from build123d import *

# Parameters (mm, degrees)
SKETCH_1_W          = 110
SKETCH_1_H          = 85.2
EXTRUDE_1_DEPTH     = 4
SKETCH_2_W          = 83
SKETCH_2_H          = 11
CUT_EXTRUDE_1_DEPTH = 4
SKETCH_3_R          = 1.6
CUT_EXTRUDE_2_DEPTH = 4
FILLET_1_R          = 2


with BuildPart() as part:
    # 草图1 → 凸台-拉伸1 (new body)
    with BuildSketch(Plane(origin=(0, 0, 0), x_dir=(1, 0, 0), z_dir=(0, 1, 0))):
        Rectangle(SKETCH_1_W, SKETCH_1_H)
    extrude(amount=EXTRUDE_1_DEPTH)

    # 草图2 → 切除-拉伸1 (cut)
    with BuildSketch(Plane(origin=(0, 4, 0), x_dir=(1, 0, 0), z_dir=(0, 1, 0))):
        with Locations((-55, -42.6)):
            Rectangle(SKETCH_2_W, SKETCH_2_H)
        with Locations((55, -42.6)):
            Rectangle(SKETCH_2_W, SKETCH_2_H)
        with Locations((55, 42.6)):
            Rectangle(SKETCH_2_W, SKETCH_2_H)
        with Locations((-55, 42.6)):
            Rectangle(SKETCH_2_W, SKETCH_2_H)
    extrude(amount=-CUT_EXTRUDE_1_DEPTH, mode=Mode.SUBTRACT)

    # 草图3 → 切除-拉伸2 (cut)
    with BuildSketch(Plane(origin=(0, 4, 0), x_dir=(1, 0, 0), z_dir=(0, 1, 0))):
        with Locations(Location((-8, -39.85, 0), (0, 0, 270))):
            Circle(SKETCH_3_R)
        with Locations(Location((8, -39.85, 0), (0, 0, 90))):
            Circle(SKETCH_3_R)
        with Locations(Location((8, 39.85, 0), (0, 0, 270))):
            Circle(SKETCH_3_R)
        with Locations(Location((-8, 39.85, 0), (0, 0, 90))):
            Circle(SKETCH_3_R)
    extrude(amount=-CUT_EXTRUDE_2_DEPTH, mode=Mode.SUBTRACT)

    # 圆角1
    fillet_1_edges = [part.edges().sort_by_distance(p)[0] for p in [
        (-13.5, 2, 42.6),
        (-13.5, 2, 37.1),
        (-55, 2, 37.1),
        (13.5, 2, 42.6),
        (55, 2, 37.1),
        (13.5, 2, 37.1),
        (55, 2, -37.1),
        (13.5, 2, -42.6),
        (13.5, 2, -37.1),
        (-13.5, 2, -42.6),
        (-55, 2, -37.1),
        (-13.5, 2, -37.1),
    ]]
    fillet(fillet_1_edges, radius=FILLET_1_R)


solid = part.part
The model under review builds one solid part; all positions refer to its coordinate system, in mm. A direction names the side the tool comes from. Coordinates: 2 decimals unless noted, no trailing zeros. Loops run counter-clockwise (first coordinate to the right, second up) from the corner with the lowest first, then second, coordinate; pieces in that order, holes last.
(1) Draft analysis for pull direction Z (two halves, no side actions). For faces 5 (the cylindrical face through (-9.56, 2.03, 39.5)), 6 (the flat face through (0, 2, -42.6)), 7 (the flat face through (0, 2, 42.6)), 8 (the flat face through (-1, 4, -1)), state which applies: +Z half, -Z half, draft (parallel to the pull), parting line (faces both ways), or undercut.
Determined:
face 5: undercut
face 6: -Z half
face 7: +Z half
face 8: draft
(2) Tool access review of faces 1 (the flat face through (-35, 2, 37.1)), 2 (the flat face through (-35, 2, -37.1)), 3 (the flat face through (34, 2, 37.1)), 4 (the flat face through (34, 2, -37.1)): name each direction out of +Z, -Z, +X, -X, +Y, -Y from which nothing blocks a thin tool from reaching the whole face with its end or side.
Determined:
face 1: +Z, -X, +Y, -Y
face 2: -Z, -X, +Y, -Y
face 3: +Z, +X, +Y, -Y
face 4: -Z, +X, +Y, -Y
(3) Consider section A-A, the plane x = 8. Give the boundary of the cut face in (y, z), plus the area to 3 significant figures.
Determined:
outline: (0, -42.6) - (4, -42.6) - (4, -41.45) - (0, -41.45) - close; (0, -38.25) - (4, -38.25) - (4, 38.25) - (0, 38.25) - close; (0, 41.45) - (4, 41.45) - (4, 42.6) - (0, 42.6) - close
area: 315 mm2
(4) Consider section C-C, the plane x = -28. Give the boundary of the cut face in (y, z), plus the area to 3 significant figures.
Determined:
outline: (0, -37.1) - (4, -37.1) - (4, 37.1) - (0, 37.1) - close
area: 297 mm2
(5) Consider section B-B, the plane y = 1.45. Give the boundary of the cut face in (x, z), plus the area to 3 significant figures.
Determined:
outline: (-55, -35.1) arc R2 ccw to (-53, -37.1) - (-15.5, -37.1) arc R2 cw to (-13.5, -39.1) - (-13.5, -40.6) arc R2 ccw to (-11.5, -42.6) - (11.5, -42.6) arc R2 ccw to (13.5, -40.6) - (13.5, -39.1) arc R2 cw to (15.5, -37.1) - (53, -37.1) arc R2 ccw to (55, -35.1) - (55, 35.1) arc R2 ccw to (53, 37.1) - (15.5, 37.1) arc R2 cw to (13.5, 39.1) - (13.5, 40.6) arc R2 ccw to (11.5, 42.6) - (-11.5, 42.6) arc R2 ccw to (-13.5, 40.6) - (-13.5, 39.1) arc R2 cw to (-15.5, 37.1) - (-53, 37.1) arc R2 ccw to (-55, 35.1) - close; hole circle Ø3.2 at (-8, -39.85); hole circle Ø3.2 at (-8, 39.85); hole circle Ø3.2 at (8, -39.85); hole circle Ø3.2 at (8, 39.85)
area: 8,420 mm2
(6) Insertion check: P1, Ø1.2, axis at x = 29, y = 2, coming from the +Z side; P2, Ø1.5, axis at x = -27, y = 2.5, coming from the -Z side; P3, Ø1.6, axis at y = 1.5, z = -40, coming from the +X side; P4, Ø3.5, axis at x = -8, z = 39.85, coming from the -Y side. Each pin has a flat end and moves straight along its axis. Give the tip position at first contact, or say it passes through.
Determined:
P1: stops at z = 37.1
P2: stops at z = -37.1
P3: stops at x = 13.5
P4: stops at y = 0
(7) Wall thickness on L1, parallel to X at y = 1.5, z = 39.85; L2, parallel to Z at x = 27, y = 2.9; L3, parallel to X at y = 3.6, z = 38: over which ranges is each line inside the solid? List them lowest first.
Determined:
L1: x = -13.5 to -9.6, -6.4 to 6.4, 9.6 to 13.5
L2: z = -37.1 to 37.1
L3: x = -13.83 to 13.83
